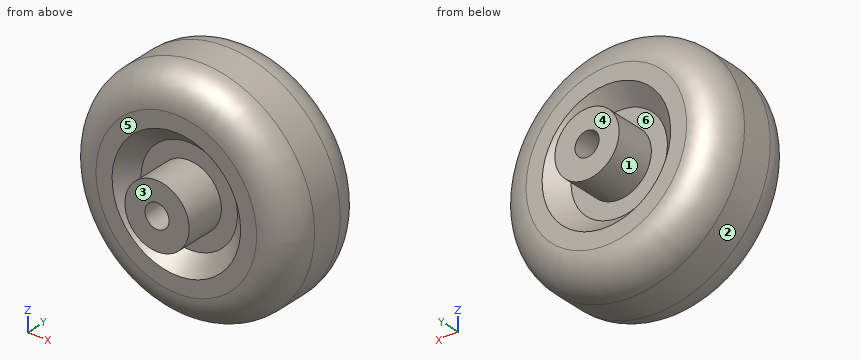
```python
from build123d import *

# Parameters (mm, degrees)
F3_D = 19.05
F4_R = 25.4


with BuildPart() as f1:
    # F0 (on Right) → F1 (revolve)
    with BuildSketch(Plane.YZ):
        Polygon((0, 25.4), (0, 0), (114.3, 0), (114.3, 25.4), (82.55, 25.4), (82.55, 38.1), (95.25, 50.8), (95.25, 88.9), (19.05, 88.9), (19.05, 50.8), (31.75, 38.1), (31.75, 25.4), align=None)
    revolve(axis=Axis((0, 77.023387, 0), (0, 1, 0)))

    # F3 (through all)
    with Locations(Plane(origin=(0, 114.3, 0), x_dir=(-1, 0, 0), z_dir=(0, 1, 0))):
        with Locations((0, 0)):
            Hole(F3_D / 2)

    # F4
    f4_edges = [f1.edges().sort_by_distance(p)[0] for p in [
        (0, 95.25, -88.9),
        (0, 19.05, -88.9),
    ]]
    fillet(f4_edges, radius=F4_R)


solid = f1.part
```
Design review of the part built by this model. Coordinates are the model's own, in mm. Face numbers are marked on the shaded views. A direction names the side the tool comes from. Give positions to 0.01 mm unless a question says otherwise; leave off trailing zeros. Loops run counter-clockwise (first coordinate to the right, second up) from the corner with the lowest first, then second, coordinate; pieces in that order, holes last. Notation, with made-up numbers: M 9,-17.75 L 16,-17.75 A19 ccw 16,-9.75 Z; hole C 60,23.5 d5. An arc over 180 degrees is marked long. Return JSON: item names as keys, results as strings. Group by question number.
Item 1: We need section A-A (z = 0). Give the boundary of the cut face in (x, y) (3 decimals).
Item 2: Insertion check: pin 1 Ø8 at (x, y) = (18.5, 74.5) entering from -Z; pin 2 Ø1.5 at (y, z) = (82.5, -16) entering from +X; pin 3 Ø5 at (x, z) = (-27, -34) entering from +Y. Each pin has a flat end and moves straight along its axis. Give the tip position at first contact, or say it passes through.
Item 3: We need section B-B (x = 0). Give the boundary of the cut face in (y, z) (3 decimals).
Item 4: Mouldability with a two-part tool opening along X and no side actions: class the marked faces 1, 2 and 3 as released by +X, released by -X, zero draft, split by the parting line, or undercut.
Item 5: For probe 1 along Y at (x, z) = (-14.5, -62); probe 2 along Y at (x, z) = (-23, -14); probe 3 along Z at (x, y) = (26, 24), list the stretches that pass through material, from the lowest coordinate up.
Item 6: Tool access review of the marked faces 4, 5 and 6: name each direction out of +Z, -Z, +X, -X, +Y, -Y from which nothing blocks a thin tool from reaching the whole face with its end or side.
Item 7: We need section D-D (y = 41). Give the boundary of the cut face in (x, z) (3 decimals), and give its area (3 significant figures).
Item 8: We need section C-C (y = 87.5). Give the number of separate pieces and of enclosed holes in the cut face, and give its area (3 significant figures).
Output:
{
 "1": {"outline": "M -88.9,44.45 A25.4 ccw -63.5,19.05 L -50.8,19.05 L -38.1,31.75 L -25.4,31.75 L -25.4,0 L -9.525,0 L -9.525,114.3 L -25.4,114.3 L -25.4,82.55 L -38.1,82.55 L -50.8,95.25 L -63.5,95.25 A25.4 ccw -88.9,69.85 Z; M 9.525,0 L 25.4,0 L 25.4,31.75 L 38.1,31.75 L 50.8,19.05 L 63.5,19.05 A25.4 ccw 88.9,44.45 L 88.9,69.85 A25.4 ccw 63.5,95.25 L 50.8,95.25 L 38.1,82.55 L 25.4,82.55 L 25.4,114.3 L 9.525,114.3 Z"},
 "2": {"pin 1": "stops at z = -87.48", "pin 2": "stops at x = 84.46", "pin 3": "stops at y = 90.37"},
 "3": {"outline": "M 0,-25.4 L 31.75,-25.4 L 31.75,-38.1 L 19.05,-50.8 L 19.05,-63.5 A25.4 ccw 44.45,-88.9 L 69.85,-88.9 A25.4 ccw 95.25,-63.5 L 95.25,-50.8 L 82.55,-38.1 L 82.55,-25.4 L 114.3,-25.4 L 114.3,-9.525 L 0,-9.525 Z; M 0,9.525 L 114.3,9.525 L 114.3,25.4 L 82.55,25.4 L 82.55,38.1 L 95.25,50.8 L 95.25,63.5 A25.4 ccw 69.85,88.9 L 44.45,88.9 A25.4 ccw 19.05,63.5 L 19.05,50.8 L 31.75,38.1 L 31.75,25.4 L 0,25.4 Z"},
 "4": {"face 1": "undercut", "face 2": "split by the parting line", "face 3": "zero draft"},
 "5": {"probe 1": "y = 19.05 to 95.25", "probe 2": "y = 31.75 to 82.55", "probe 3": "z = -74.14 to -37.77, 37.77 to 74.14"},
 "6": {"face 4": "+Z, -Z, +X, -X, +Y", "face 5": "-Y", "face 6": "+Y"},
 "7": {"outline": "C 0,0 d177.329; hole C 0,0 d19.05", "area": "24,400 mm^2"},
 "8": {"separate pieces": "2", "enclosed holes": "2", "area": "16,900 mm^2"}
}
